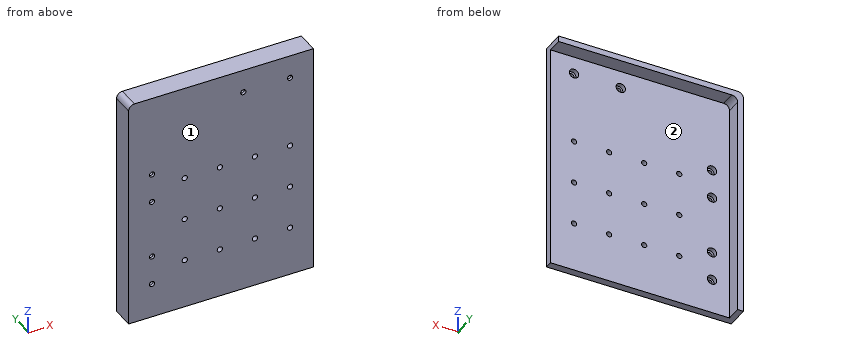
```python
from build123d import *

# Parameters (mm, degrees)
SKETCH1_W                      = 158
SKETCH1_H                      = 199.5
BOSS_EXTRUDE1_DEPTH            = 6.35
BOSS_EXTRUDE2_DEPTH            = 12.7
CBORE_FOR_M4_SHCS1_D           = 4.5
CBORE_FOR_M4_SHCS1_DEPTH       = 6.35
CBORE_FOR_M4_SHCS1_CBORE_D     = 8
CBORE_FOR_M4_SHCS1_CBORE_DEPTH = 4
M4_CLEARANCE_HOLE2_D           = 4.5
M4_CLEARANCE_HOLE2_DEPTH       = 6.35
LPATTERN1_COUNT                = 4
LPATTERN1_PITCH                = 30
LPATTERN1_COUNT_DIR2           = 3
LPATTERN1_PITCH_DIR2           = 37.5
FILLET2_R                      = 5


with BuildPart() as part:
    # Sketch1 → Boss-Extrude1 (new body)
    with BuildSketch(Plane(origin=(0, 0, 0), x_dir=(1, 0, 0), z_dir=(0, 1, 0))):
        with Locations((79, -99.75)):
            Rectangle(SKETCH1_W, SKETCH1_H)
    extrude(amount=BOSS_EXTRUDE1_DEPTH)

    # Sketch3 → Boss-Extrude2 (add)
    with BuildSketch(Plane(origin=(0, 6.35, 0), x_dir=(1, 0, 0), z_dir=(0, 1, 0))):
        Polygon((0, 0), (0, -199.5), (158, -199.5), (158, -194.5), (5, -194.5), (5, 0), align=None)
    extrude(amount=BOSS_EXTRUDE2_DEPTH)

    # CBORE for M4 SHCS1
    with Locations(Plane(origin=(0, 6.35, 0), x_dir=(1, 0, 0), z_dir=(0, 1, 0))):
        with Locations((20, -55), (98, -179.5), (138, -179.5), (20, -130), (20, -105), (20, -30)):
            CounterBoreHole(CBORE_FOR_M4_SHCS1_D / 2, CBORE_FOR_M4_SHCS1_CBORE_D / 2, CBORE_FOR_M4_SHCS1_CBORE_DEPTH, depth=CBORE_FOR_M4_SHCS1_DEPTH)

    # M4 Clearance Hole2
    with Locations(Plane(origin=(0, 6.35, 0), x_dir=(1, 0, 0), z_dir=(0, 1, 0))):
        with Locations((138, -117.5)):
            m4_clearance_hole2 = Hole(M4_CLEARANCE_HOLE2_D / 2, depth=M4_CLEARANCE_HOLE2_DEPTH)

    # LPattern1: M4 Clearance Hole2 4 × 3
    with Locations(*[(-i * LPATTERN1_PITCH, 0, -j * LPATTERN1_PITCH_DIR2) for i in range(LPATTERN1_COUNT) for j in range(LPATTERN1_COUNT_DIR2) if (i, j) != (0, 0)]):
        add(m4_clearance_hole2, mode=Mode.SUBTRACT)

    # Fillet2
    fillet2_edges = [part.edges().sort_by_distance(p)[0] for p in [
        (5, 12.7, 194.5),
        (0, 9.525, 199.5),
    ]]
    fillet(fillet2_edges, radius=FILLET2_R)


solid = part.part
```
Work out the finished part from the listing and answer in its coordinate system (mm). Face numbers are marked on the shaded views. A direction names the side the tool comes from. Coordinates: 2 decimals unless noted, no trailing zeros. Order: outer loops, then holes, each group sorted by start corner. A loop starts at its lowest first (then second) coordinate and runs counter-clockwise, first axis right, second up. Notation, with made-up numbers: (38, 23.5) - (84, 23.5) arc R27 cw to (84, 50.5) - close; hole circle Ø4 at (-8.75, 79). An arc over 180 degrees is marked (long way). Answer as a JSON object with one key per item and string values.
1. Each of these flat-tipped pins is pushed along its axis until it touches: P1, Ø6, axis at y = 16.5, z = 131, coming from the +X side; P2, Ø12, axis at x = 91, z = 178, coming from the +Y side; P3, Ø6.5, axis at x = 20, z = 130, coming from the +Y side. Where does it stop, or does it pass through?
Output values:
{"P1": "stops at x = 5", "P2": "stops at y = 6.35", "P3": "stops at y = 2.35"}
2. Find section C-C on z = 80. Determine the outline of the cut face in (x, y), plus the area to 4 significant figures.
Output values:
{"outline": "(0, 0) - (45.75, 0) - (45.75, 6.35) - (5, 6.35) - (5, 19.05) - (0, 19.05) - close; (50.25, 0) - (75.75, 0) - (75.75, 6.35) - (50.25, 6.35) - close; (80.25, 0) - (105.75, 0) - (105.75, 6.35) - (80.25, 6.35) - close; (110.25, 0) - (135.75, 0) - (135.75, 6.35) - (110.25, 6.35) - close; (140.25, 0) - (158, 0) - (158, 6.35) - (140.25, 6.35) - close", "area": "952.5 mm²"}
3. Find section A-A on z = 30. Determine the outline of the cut face in (x, y).
Output values:
{"outline": "(0, 0) - (17.75, 0) - (17.75, 2.35) - (16, 2.35) - (16, 6.35) - (5, 6.35) - (5, 19.05) - (0, 19.05) - close; (22.25, 0) - (158, 0) - (158, 6.35) - (24, 6.35) - (24, 2.35) - (22.25, 2.35) - close"}
4. Consider line 1 (Z direction, x = 78, y = 2.25); line 2 (Z direction, x = 138, y = 3.25); line 3 (Z direction, x = 20, y = 0.5). Determine where each line is inside the solid, lowest interval first.
Output values:
{"line 1": "z = 0 to 40.25, 44.75 to 77.75, 82.25 to 115.25, 119.75 to 199.5", "line 2": "z = 0 to 40.25, 44.75 to 77.75, 82.25 to 115.25, 119.75 to 175.5, 183.5 to 199.5", "line 3": "z = 0 to 27.75, 32.25 to 52.75, 57.25 to 102.75, 107.25 to 127.75, 132.25 to 199.5"}
5. Find section B-B on x = 108. Determine the outline of the cut face in (y, z).
Output values:
{"outline": "(0, 0) - (6.35, 0) - (6.35, 40.25) - (0, 40.25) - close; (0, 44.75) - (6.35, 44.75) - (6.35, 77.75) - (0, 77.75) - close; (0, 82.25) - (6.35, 82.25) - (6.35, 115.25) - (0, 115.25) - close; (0, 119.75) - (6.35, 119.75) - (6.35, 194.5) - (19.05, 194.5) - (19.05, 199.5) - (0, 199.5) - close"}
6. Find section D-D on x = 138. Determine the outline of the cut face in (y, z).
Output values:
{"outline": "(0, 0) - (6.35, 0) - (6.35, 40.25) - (0, 40.25) - close; (0, 44.75) - (6.35, 44.75) - (6.35, 77.75) - (0, 77.75) - close; (0, 82.25) - (6.35, 82.25) - (6.35, 115.25) - (0, 115.25) - close; (0, 119.75) - (6.35, 119.75) - (6.35, 175.5) - (2.35, 175.5) - (2.35, 177.25) - (0, 177.25) - close; (0, 181.75) - (2.35, 181.75) - (2.35, 183.5) - (6.35, 183.5) - (6.35, 194.5) - (19.05, 194.5) - (19.05, 199.5) - (0, 199.5) - close"}
7. A tool of negligible diameter and unlimited length cuts with its end or side. For the marked faces 1 and 2, from which of +Z, -Z, +X, -X, +Y, -Y can it reach the whole face along a straight path? Write none if from no direction.
Output values:
{"face 1": "+Z, -Z, +X, -X, -Y", "face 2": "-Z, +X, +Y"}
